Could you check a few things on this model? Use its own coordinates, in mm. Face numbers are marked on the shaded views. Round coordinates to 2 decimals unless told otherwise and drop trailing zeros. Loops run counter-clockwise (first coordinate to the right, second up) from the corner with the lowest first, then second, coordinate; pieces in that order, holes last. Notation, with made-up numbers: (34, 74.5) -> (52, 74.5) arc R10 cw to (52, 86.5) -> close; hole circle Ø1 at (22.25, 53.5). An arc over 180 degrees is marked (long way). Write each question's results on one line, items separated by ' | '. Start each with the question number.
1) For P1, Ø0.8, axis at x = 587.5, y = 26.5, coming from the +Z side; P2, Ø3, axis at y = 27, z = -739, coming from the +X side; P3, Ø0.8, axis at y = 27, z = -590.5, coming from the -X side, each with a flat end and sliding along its axis, tell me the tip position at first contact or that it passes through.
2) Imagine slicing it at A-A, the plane z = -1588.5. List the corners of the cut face in (x, y) for me, plus the area to 3 significant figures.
3) If I drill on probe 1 along X at (y, z) = (26.25, -577); probe 2 along Y at (x, z) = (630.5, -117); probe 3 along Z at (x, y) = (1637.5, 26.5), over which ranges is the centre line in solid material (lowest first)?
4) We'd pull the mould along X, two halves only. Please class the marked faces 1, 2 and 3: pulls with the +X half, pulls with the -X half, needs draft (parallel to the pull), parting line crosses it, or undercut.
5) Imagine slicing it at B-B, the plane x = 81. List the corners of the cut face in (y, z) for me.
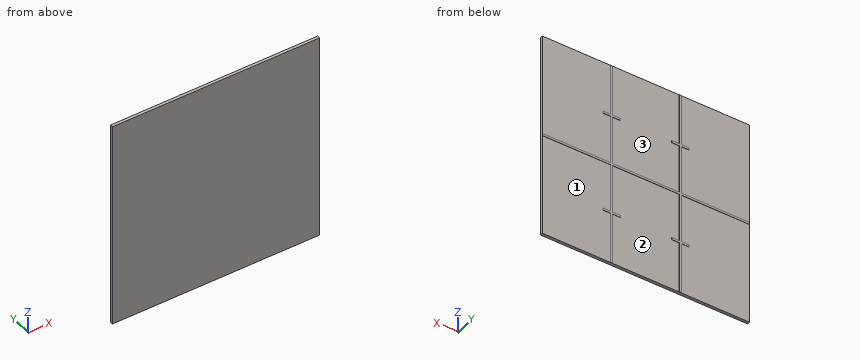
from build123d import *

# Parameters (mm, degrees)
SKETCH1_W           = 1828.8
SKETCH1_H           = 1828.8
BOSS_EXTRUDE1_DEPTH = 25.4
BOSS_EXTRUDE2_DEPTH = 2.54


with BuildPart() as part:
    # Sketch1 → Boss-Extrude1 (new body)
    with BuildSketch(Plane(origin=(0, 0, 0), x_dir=(1, 0, 0), z_dir=(0, 1, 0))):
        with Locations((850.696210424, 904.080811624)):
            Rectangle(SKETCH1_W, SKETCH1_H)
    extrude(amount=BOSS_EXTRUDE1_DEPTH)

    # Sketch2 → Boss-Extrude2 (add)
    with BuildSketch(Plane(origin=(0, 25.4, 0), x_dir=(1, 0, 0), z_dir=(0, 1, 0))):
        Polygon((1765.096210424, 913.605811624), (1765.096210424, 894.555811624), (1165.021210424, 894.555811624), (1165.021210424, 463.924675702), (1230.050709734, 463.924675702), (1230.050709734, 444.874675702), (1165.021210424, 444.874675702), (1165.021210424, -10.319188376), (1145.971210424, -10.319188376), (1145.971210424, 444.874675702), (1077.650709734, 444.874675702), (1077.650709734, 463.924675702), (1145.971210424, 463.924675702), (1145.971210424, 894.555811624), (557.066711115, 894.555811624), (557.066711115, 463.924675702), (623.741711115, 463.924675702), (623.741711115, 444.874675702), (557.066711115, 444.874675702), (557.066711115, -10.319188376), (538.016711115, -10.319188376), (538.016711115, 444.874675702), (471.341711115, 444.874675702), (471.341711115, 463.924675702), (538.016711115, 463.924675702), (538.016711115, 894.555811624), (-63.703789576, 894.555811624), (-63.703789576, 913.605811624), (538.016711115, 913.605811624), (538.016711115, 1344.236947546), (471.341711115, 1344.236947546), (471.341711115, 1363.286947546), (538.016711115, 1363.286947546), (538.016711115, 1818.480811624), (557.066711115, 1818.480811624), (557.066711115, 1363.286947546), (623.741711115, 1363.286947546), (623.741711115, 1344.236947546), (557.066711115, 1344.236947546), (557.066711115, 913.605811624), (1145.971210424, 913.605811624), (1145.971210424, 1344.236947546), (1077.650709734, 1344.236947546), (1077.650709734, 1363.286947546), (1145.971210424, 1363.286947546), (1145.971210424, 1818.480811624), (1155.496210424, 1818.480811624), (1165.021210424, 1818.480811624), (1165.021210424, 1363.286947546), (1230.050709734, 1363.286947546), (1230.050709734, 1344.236947546), (1165.021210424, 1344.236947546), (1165.021210424, 913.605811624), align=None)
    extrude(amount=BOSS_EXTRUDE2_DEPTH)


solid = part.part
Checked values:
1) P1: z = -444.87 | P2: x = 1165.02 | P3: x = 538.02
2) outline: (-63.7, 0) -> (1765.1, 0) -> (1765.1, 25.4) -> (1165.02, 25.4) -> (1165.02, 27.94) -> (1145.97, 27.94) -> (1145.97, 25.4) -> (557.07, 25.4) -> (557.07, 27.94) -> (538.02, 27.94) -> (538.02, 25.4) -> (-63.7, 25.4) -> close | area: 46,500 mm^2
3) probe 1: 538.02 to 557.07, 1145.97 to 1165.02 | probe 2: 0 to 25.4 | probe 3: -913.61 to -894.56
4) face 1: needs draft | face 2: undercut | face 3: undercut
5) outline: (0, -1818.48) -> (25.4, -1818.48) -> (25.4, -913.61) -> (27.94, -913.61) -> (27.94, -894.56) -> (25.4, -894.56) -> (25.4, 10.32) -> (0, 10.32) -> close
